Autodesk Inventor part; units mm, degrees
ref_plane "YZ Plane" through (0, 0, 0) normal (1, 0, 0) x (0, 1, 0)
ref_plane "XZ Plane" through (0, 0, 0) normal (0, 1, 0) x (-1, 0, 0)
ref_plane "XY Plane" through (0, 0, 0) normal (0, 0, 1) x (1, 0, 0)
sketch "Sketch1" plane through (0, 0, 0) normal (0, 1, 0) x (-1, 0, 0)
  circle A0 centre (0, 0) radius 220
  dimension "d0" = 440
extrude "Extrusion1" add sketch "Sketch1" along normal blind 3.5
sketch "Sketch2" plane through (0, 3.5, 0) normal (0, 1, 0) x (1, 0, 0)
  line L0 (-66.25, 171.8) -> (66.25, 171.8)
  line L1 (66.25, 171.8) -> (66.25, 220)
  line L2 (66.25, 220) -> (-66.25, 220)
  line L3 (-66.25, 220) -> (-66.25, 171.8)
  circle A0 centre (0, 0) radius 220
  point P0 (0, 220)
  dimension "d3" = 132.5
  dimension "d4" = 48.2
  dimension "d5" = 0
  dimension "d6" = 220
extrude "Extrusion2" cut sketch "Sketch2" against normal through all contours L3 A0 L1 L0 | L3 L2 A0 | A0 L2 L1 picked at (0, 187.8667)
fillet "Fillet1" radius 2 4 edges at (-66.25, 1.75, -171.8) (-66.25, 1.75, -209.7878) (66.25, 1.75, -209.7878) (66.25, 1.75, -171.8)
mirror "Mirror1" about plane through (0, 0, 0) normal (0, 0, 1) of "Extrusion2", "Fillet1"
sketch "Sketch3" plane through (0, 3.5, 0) normal (0, 1, 0) x (1, 0, 0)
  line L0 (0, 0) -> (-120, 0)
  line L1 (-120, 0) -> (-120, 155)
  circle A0 centre (-120, 155) radius 2.25
  circle A1 centre (120, 155) radius 2.25
  circle A2 centre (-120, -155) radius 2.25
  circle A3 centre (120, -155) radius 2.25
  dimension "d10" = 120
  dimension "d11" = 155
  dimension "d12" = 4.5
  dimension "d15" = 240
  dimension "d18" = 310
extrude "Extrusion3" cut sketch "Sketch3" against normal blind 10
properties part number "AMR_base" material "Aluminum 6061"
Input: part model. Units: mm. Frame: model coordinates. Give positions to 0.01 mm unless a question says otherwise; leave off trailing zeros. Loops run counter-clockwise (first coordinate to the right, second up) from the corner with the lowest first, then second, coordinate; pieces in that order, holes last. Notation, with made-up numbers: (44.5, 31) -> (68.5, 31) arc R17 ccw to (68.5, 51) -> close; hole circle Ø9 at (-22.75, 14). An arc over 180 degrees is marked (long way). Answer as a JSON object with one key per item and string values. Group by question number.
Item 1: Cut plane C-C, the plane z = 71. Return the cut outline in (x, y), and give its area (3 significant figures).
Item 2: Line query: probe 1 along X at (y, z) = (2.05, 155); probe 2 along Z at (x, y) = (-120, 2.65); probe 3 along Z at (x, y) = (36, 3.2). Output: solid intervals per line, ascending.
Item 3: Pin query (flat end, axial travel): P1, Ø2.5, axis at x = -120, z = 155, coming from the -Y side; P2, Ø1.8, axis at y = 1.5, z = 198.5, coming from the -X side; P3, Ø1, axis at y = 2, z = -198, coming from the +X side; P4, Ø1.8, axis at y = 2, z = -198, coming from the -X side. Return the tip coordinate at first contact, or that it passes through.
Item 4: Cut plane B-B, the plane x = 1. Return the cut outline in (y, z), and give its area (3 significant figures).
Item 5: Cut plane A-A, the plane y = 1.5. Return the cut outline in (x, z).
Checks:
{
 "1": {"outline": "(-208.23, 0) -> (208.23, 0) -> (208.23, 3.5) -> (-208.23, 3.5) -> close", "area": "1,460 mm²"},
 "2": {"probe 1": "x = -156.12 to -122.25, -117.75 to 117.75, 122.25 to 156.12", "probe 2": "z = -184.39 to -157.25, -152.75 to 152.75, 157.25 to 184.39", "probe 3": "z = -171.8 to 171.8"},
 "3": {"P1": "passes through", "P2": "stops at x = -96.72", "P3": "stops at x = 96.92", "P4": "stops at x = -97.73"},
 "4": {"outline": "(0, -171.8) -> (3.5, -171.8) -> (3.5, 171.8) -> (0, 171.8) -> close", "area": "1,200 mm²"},
 "5": {"outline": "(-68.88, -208.94) arc R2 ccw to (-66.25, -207.04) -> (-66.25, -173.8) arc R2 cw to (-64.25, -171.8) -> (64.25, -171.8) arc R2 cw to (66.25, -173.8) -> (66.25, -207.04) arc R2 ccw to (68.88, -208.94) arc R220 ccw to (68.88, 208.94) arc R2 ccw to (66.25, 207.04) -> (66.25, 173.8) arc R2 cw to (64.25, 171.8) -> (-64.25, 171.8) arc R2 cw to (-66.25, 173.8) -> (-66.25, 207.04) arc R2 ccw to (-68.88, 208.94) arc R220 ccw to start; hole circle Ø4.5 at (-120, -155); hole circle Ø4.5 at (-120, 155); hole circle Ø4.5 at (120, -155); hole circle Ø4.5 at (120, 155)"}
}
